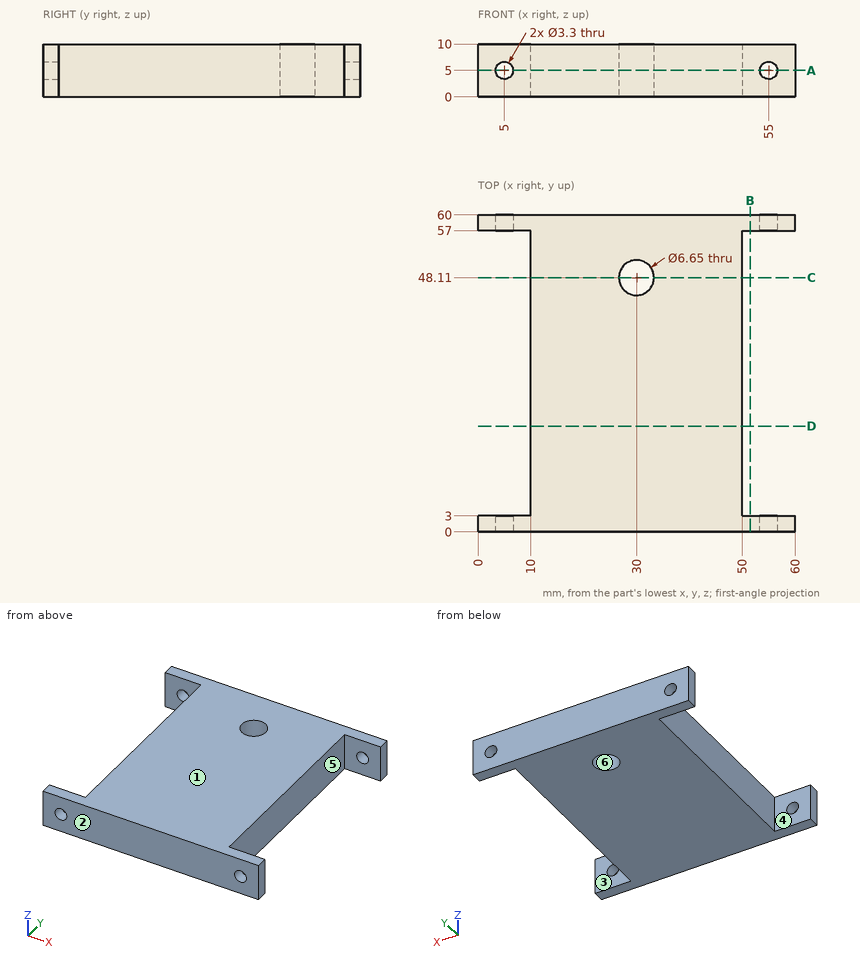
Could you check a few things on this drawing? It's one solid part, dimensions in mm from its lowest x, y, z. A direction names the side the tool comes from. Give positions to 0.01 mm unless a question says otherwise; leave off trailing zeros. Order: outer loops, then holes, each group sorted by start corner. A loop starts at its lowest first (then second) coordinate and runs counter-clockwise, first axis right, second up. Notation, with made-up numbers: (57, 71) - (82, 71) arc R6 cw to (82, 80) - close; hole circle Ø7 at (5.25, -13.75). An arc over 180 degrees is marked (long way). Return JSON: item names as keys, results as strings. Group by question number.
Q1. Please list where these lines run through material, in increasing order: line 1 along Y through (x, z) = (8, 5.25); line 2 along Z through (x, y) = (55, 1.15); line 3 along Y through (x, z) = (30, 4.75) (3 decimals). Write a range as [from, to].
Q2. Suppose I cut it at B-B, the plane x = 51.5. Please give me the cut outline in (y, z).
Q3. Thinking about a two-plate mould opening in Y: for the marked faces 1, 2 and 3, which applies, pulls with the +Y half, pulls with the -Y half, needs draft (parallel to the pull), parting line crosses it, or undercut?
Q4. Suppose I cut it at C-C, the plane y = 48.11. Please give me the cut outline in (x, z) (3 decimals), and give its area (4 significant figures).
Q5. Will these pins go through, and if not, where does the flat tip stop? pin 1 Ø6 at (y, z) = (45.5, 3.5) entering from +X; pin 2 Ø5 at (y, z) = (23, 1.5) entering from -X.
Q6. Which directions (+Z, -Z, +X, -X, +Y, -Y) give clear straight access to the entire face, cutting with the end or side of a thin tool? Please do the marked faces 4, 5 and 6.
Q7. Suppose I cut it at D-D, the plane y = 20. Please give me the cut outline in (x, z).
Q8. Suppose I cut it at A-A, the plane z = 5. State how many separate pieces and enclosed holes the cut face has, and give its area (3 significant figures).
Resolved:
{
 "1": {"line 1": "y = [0, 3], [57, 60]", "line 2": "z = [0, 3.35], [6.65, 10]", "line 3": "y = [0, 44.785], [51.435, 60]"},
 "2": {"outline": "(0, 0) - (3, 0) - (3, 10) - (0, 10) - close; (57, 0) - (60, 0) - (60, 10) - (57, 10) - close"},
 "3": {"face 1": "needs draft", "face 2": "pulls with the -Y half", "face 3": "undercut"},
 "4": {"outline": "(10, 0) - (26.675, 0) - (26.675, 10) - (10, 10) - close; (33.325, 0) - (50, 0) - (50, 10) - (33.325, 10) - close", "area": "333.5 mm2"},
 "5": {"pin 1": "stops at x = 50", "pin 2": "stops at x = 10"},
 "6": {"face 4": "+Z, -Z, -X", "face 5": "+Z, -Z, +X", "face 6": "+Z, -Z"},
 "7": {"outline": "(10, 0) - (50, 0) - (50, 10) - (10, 10) - close"},
 "8": {"separate pieces": "5", "enclosed holes": "1", "area": "2,450 mm2"}
}
